```python
from build123d import *

# Parameters (mm, degrees)
CUT_EXTRUDE1_DEPTH      = 38.5
CUT_EXTRUDE1_DEPTH_BACK = 38.5
SKETCH2_OUTSIDE_W       = 39.248
SKETCH2_OUTSIDE_H       = 39.248
SKETCH11_W              = 30.3
SKETCH11_H              = 2.599351838
BOSS_EXTRUDE2_DEPTH     = 10
CUT_EXTRUDE6_DEPTH      = 45.205596297
CUT_EXTRUDE6_DEPTH_BACK = 45.205596297
SKETCH13_W              = 18.3
SKETCH13_H              = 8
CUT_EXTRUDE7_DEPTH      = 30.719750749
SKETCH14_R              = 2
CUT_EXTRUDE8_DEPTH      = 30.719750749
CHAMFER1_SIZE           = 2


with BuildPart() as part:
    # Sketch1 → Revolve1 (revolve)
    with BuildSketch(Plane.XY, mode=Mode.PRIVATE) as revolve1_sk:
        Polygon((15.15, 0), (25, 9.85), (25, 10.85), (22.5, 10.85), (22.5, 10.885533906), (14.114466094, 2.5), (-14.114466094, 2.5), (-22.5, 10.885533906), (-22.5, 10.85), (-25, 10.85), (-25, 9.85), (-15.15, 0), align=None)
    revolve(revolve1_sk.sketch.rotate(Axis((-0.079113924, 12.5, 0), (1, 0, 0)), 270), axis=Axis((-0.079113924, 12.5, 0), (1, 0, 0)))

    # Sketch2 outside → Cut-Extrude1 (cut, two sides: drawn at the far end of the back side and taken through both)
    with BuildSketch(Plane(origin=(0, 0, 0), x_dir=(0, 0, -1), z_dir=(1, 0, 0)).offset(-CUT_EXTRUDE1_DEPTH_BACK)):
        with Locations((0, 12.5)):
            Rectangle(SKETCH2_OUTSIDE_W, SKETCH2_OUTSIDE_H)
        with BuildLine():
            Line((-3.059956427, 12.5), (-3.059956427, 0.380319036))
            ThreePointArc((-3.059956427, 0.380319036), (0, 0), (3.059956427, 0.380319036))
            Line((3.059956427, 0.380319036), (3.059956427, 12.5))
            ThreePointArc((3.059956427, 12.5), (0, 15.559956427), (-3.059956427, 12.5))
        make_face(mode=Mode.SUBTRACT)
    extrude(amount=CUT_EXTRUDE1_DEPTH + CUT_EXTRUDE1_DEPTH_BACK, mode=Mode.SUBTRACT)

    # Sketch11 → Boss-Extrude2 (add, symmetric)
    with BuildSketch(Plane.XY):
        with Locations((0, 1.679994955)):
            Rectangle(SKETCH11_W, SKETCH11_H)
    extrude(amount=BOSS_EXTRUDE2_DEPTH, both=True)

    # Sketch12 → Cut-Extrude6 (cut, two sides: drawn at the far end of the back side and taken through both)
    with BuildSketch(Plane.ZY.offset(15.15).offset(-CUT_EXTRUDE6_DEPTH_BACK)):
        with BuildLine():
            Line((-3.059956427, 0.380319036), (3.059956427, 0.380319036))
            ThreePointArc((3.059956427, 0.380319036), (0, 0), (-3.059956427, 0.380319036))
        make_face()
    extrude(amount=CUT_EXTRUDE6_DEPTH + CUT_EXTRUDE6_DEPTH_BACK, mode=Mode.SUBTRACT)

    # Sketch13 → Cut-Extrude7 (cut, through all)
    with BuildSketch(Plane(origin=(0, 2.979670874, 0), x_dir=(1, 0, 0), z_dir=(0, 1, 0))):
        Rectangle(SKETCH13_W, SKETCH13_H)
    extrude(amount=-CUT_EXTRUDE7_DEPTH, mode=Mode.SUBTRACT)

    # Sketch14 → Cut-Extrude8 (cut, through all)
    with BuildSketch(Plane(origin=(0, 2.979670874, 0), x_dir=(1, 0, 0), z_dir=(0, 1, 0))):
        with Locations(Location((11.15, -6, 0), (0, 0, 270))):
            Circle(SKETCH14_R)
        with Locations(Location((-11.15, -6, 0), (0, 0, 90))):
            Circle(SKETCH14_R)
        with Locations(Location((-11.15, 6, 0), (0, 0, 270))):
            Circle(SKETCH14_R)
        with Locations(Location((11.15, 6, 0), (0, 0, 90))):
            Circle(SKETCH14_R)
    extrude(amount=-CUT_EXTRUDE8_DEPTH, mode=Mode.SUBTRACT)

    # Chamfer1
    chamfer1_edges = [part.edges().sort_by_distance(p)[0] for p in [
        (-9.15, 1.679994955, -4),
        (9.15, 1.679994955, -4),
        (9.15, 1.679994955, 4),
        (-9.15, 1.679994955, 4),
        (15.15, 1.679994955, -10),
        (-15.15, 1.679994955, -10),
        (15.15, 1.679994955, 10),
        (-15.15, 1.679994955, 10),
    ]]
    chamfer(chamfer1_edges, length=CHAMFER1_SIZE)


solid = part.part
```
Geometry check sheet. Reference: the model listing, model coordinates, mm. A direction names the side the tool comes from. Coordinates: 2 decimals unless noted, no trailing zeros. Order: outer loops, then holes, each group sorted by start corner. A loop starts at its lowest first (then second) coordinate and runs counter-clockwise, first axis right, second up. Notation, with made-up numbers: (69.5, 56.5) - (107.5, 56.5) arc R11 cw to (107.5, 72.5) - close; hole circle Ø11 at (39.25, -4). An arc over 180 degrees is marked (long way). Use one line per item in the form item = value.
1. Section check C-C (z = 0). State how many separate pieces and enclosed holes the cut face has, then the cut area to 3 significant figures.
Here are the results:
separate_pieces = 4
enclosed_holes = 0
area = 104 mm²
2. Section check D-D (x = -10.5). Record the boundary of the cut face in (y, z), then the cut area to 3 significant figures.
Here are the results:
outline = (0.38, -10) - (2.98, -10) - (2.98, -7.89) - (0.38, -7.89) - close; (0.38, -4.11) - (2.98, -4.11) - (2.98, 4.11) - (0.38, 4.11) - close; (0.38, 7.89) - (2.98, 7.89) - (2.98, 10) - (0.38, 10) - close
area = 32.3 mm²
3. Scan lines: line 1 (X direction, y = 1.85, z = -6); line 2 (Y direction, x = 11.5, z = -9); line 3 (X direction, y = 14.25, z = 1). Record each from-to range of solid material in increasing order.
Here are the results:
line_1 = -15.15 to -13.15, -9.15 to 9.15, 13.15 to 15.15
line_2 = 0.38 to 2.98
line_3 = -25 to -22.1, 22.1 to 25
4. Section check A-A (x = 8). Record the boundary of the cut face in (y, z), then the cut area to 3 significant figures.
Here are the results:
outline = (0.38, -10) - (2.98, -10) - (2.98, -3.15) - (0.38, -3.15) - close; (0.38, 3.15) - (2.98, 3.15) - (2.98, 10) - (0.38, 10) - close
area = 35.6 mm²
5. Draft check along X on faces 1 (the face through (-22.85, 15.56, -0.07)), 2 (the face through (-25, 14, 1)), 3 (the face through (9.167, 1.698, -5.74)), 4 (the face through (-9.198, 1.698, 6.434)). Enter one of: pulls with the +X half, pulls with the -X half, needs draft (parallel to the pull), parting line crosses it, or undercut.
Here are the results:
face_1 = needs draft
face_2 = pulls with the -X half
face_3 = undercut
face_4 = undercut
6. Gauge pin test, flat ends, axial feed: pin 1 (2 mm diameter, centred on y = 1.5, z = 0.5, fed in from +X); pin 2 (6 mm diameter, centred on x = 7.5, z = 1, fed in from +Y); pin 3 (5 mm diameter, centred on x = -18.5, y = 4, fed in from +Z). Record the tip position at first contact, or that the pin passes through.
Here are the results:
pin_1 = 17.64
pin_2 = 2.98
pin_3 = 3.06
7. Section check B-B (z = -6). Record the boundary of the cut face in (x, y), then the cut area to 3 significant figures.
Here are the results:
outline = (-15.15, 0.38) - (-13.15, 0.38) - (-13.15, 2.98) - (-15.15, 2.98) - close; (-9.15, 0.38) - (9.15, 0.38) - (9.15, 2.98) - (-9.15, 2.98) - close; (13.15, 0.38) - (15.15, 0.38) - (15.15, 2.98) - (13.15, 2.98) - close
area = 58.0 mm²
8. Access from +Z, -Z, +X, -X, +Y, -Y to the whole of each face (thin tool, end or side, straight path). Record for faces 5 (the face through (0, 2, 4)), 6 (the face through (21.393, 9.786, 0.198)), 7 (the face through (-23.768, 13.964, 0.761)), 8 (the face through (-15.15, 2, -5)).
Here are the results:
face_5 = +Y, -Y
face_6 = none
face_7 = -X
face_8 = -Z, -X, +Y, -Y
